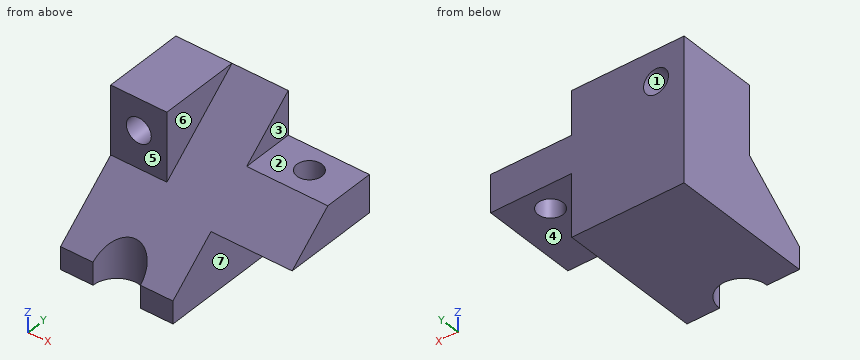
from build123d import *

# Parameters (mm, degrees)
F1_DEPTH = 77.5
F2_W     = 65
F2_H     = 35
F2_H_2   = 50
F3_DEPTH = 100
F4_R     = 19
F4_R_2   = 10
F5_DEPTH = 160.94138
F7_DEPTH = 45
F8_R     = 10
F9_DEPTH = 65


with BuildPart() as f1:
    # F0 (on Right) → F1 (new body, symmetric)
    with BuildSketch(Plane.YZ):
        Polygon((-57.5, 0), (57.5, 0), (57.5, 115), (-57.5, 18), align=None)
    extrude(amount=F1_DEPTH, both=True)

    # F2 (on Front) → F3 (cut, symmetric)
    with BuildSketch(Plane.XZ):
        with Locations((45, 97.5)):
            Rectangle(F2_W, F2_H)
        with Locations((45, 25)):
            Rectangle(F2_W, F2_H_2)
    extrude(amount=F3_DEPTH, both=True, mode=Mode.SUBTRACT)

    # F4 (on Top) → F5 (cut)
    with BuildSketch(Plane.XY):
        with Locations((-32.5, -57.5)):
            Circle(F4_R)
        with Locations((45.5, 37.5)):
            Circle(F4_R_2)
    extrude(amount=F5_DEPTH, mode=Mode.SUBTRACT)

    # F6 (on face) → F7 (join)
    with BuildSketch(Plane(origin=(-77.5, 0, 0), x_dir=(0, -1, 0), z_dir=(-1, 0, 0))):
        Polygon((7.5, 115), (-57.5, 115), (7.5, 60.1739130435), align=None)
    extrude(amount=-F7_DEPTH)

    # F8 (on face) → F9 (cut, through all)
    with BuildSketch(Plane.XZ.offset(7.5)):
        with Locations((-55, 90)):
            Circle(F8_R)
    extrude(amount=-F9_DEPTH, mode=Mode.SUBTRACT)


solid = f1.part
Input: part model. Units: mm. Frame: model coordinates. Face numbers are marked on the shaded views. A direction names the side the tool comes from. Coordinates: 2 decimals unless noted, no trailing zeros. Loops run counter-clockwise (first coordinate to the right, second up) from the corner with the lowest first, then second, coordinate; pieces in that order, holes last.
(1) Section A-A on x = -55. Return the cut outline in (y, z).
(2) Section D-D on x = 53.5. Return the cut outline in (y, z).
(3) Section C-C on z = 82.5. Return the cut outline in (x, y), then the cut area to 3 significant figures.
(4) Set-up query: the marked faces 5, 6 and 7. Return all of +Z, -Z, +X, -X, +Y, -Y with unobstructed straight access to the full face (end or side cutting, diameter ignored); none if empty.
(5) Section B-B on y = -51. Return the cut outline in (x, z).
(6) Material intervals for probe 1 along Z at (x, y) = (-55, 44.5); probe 2 along X at (y, z) = (37, 70); probe 3 along X at (y, z) = (24, 15.5), sorted ascending.
(7) Pull-direction query (Z, two-part tool) for the marked faces 1, 2, 3 and 4; classes: released by +Z, released by -Z, zero draft, split by the parting line, or undercut.
(8) First-contact query: pin 1 Ø13.5 at (x, z) = (-47.5, 77.5) entering from -Y; pin 2 Ø8 at (y, z) = (14, 11.5) entering from +X; pin 3 Ø16 at (x, z) = (-55, 90) entering from +Y; pin 4 Ø23 at (x, y) = (45.5, 37.5) entering from +Z. Flat tips, straight axial feed; report the tip coordinate or a pass-through.
Data:
1. outline: (-57.5, 0) - (57.5, 0) - (57.5, 80) - (-7.5, 80) - (-7.5, 60.17) - (-57.5, 18) - close; (-7.5, 100) - (57.5, 100) - (57.5, 115) - (-7.5, 115) - close
2. outline: (-19.56, 50) - (31.5, 50) - (31.5, 80) - (16.01, 80) - close; (43.5, 50) - (57.5, 50) - (57.5, 80) - (43.5, 80) - close
3. outline: (-77.5, -7.5) - (-61.61, -7.5) - (-61.61, 57.5) - (-77.5, 57.5) - close; (-48.39, -7.5) - (-32.5, -7.5) - (-32.5, 18.97) - (12.5, 18.97) - (12.5, 57.5) - (-48.39, 57.5) - close
3. area: 3,800 mm2
4. face 5: +Z, +X, -X, -Y
4. face 6: +Z, +X, -Y
4. face 7: -Z, +X, +Y, -Y
5. outline: (-77.5, 0) - (-50.35, 0) - (-50.35, 23.48) - (-77.5, 23.48) - close; (-14.65, 0) - (12.5, 0) - (12.5, 23.48) - (-14.65, 23.48) - close
6. probe 1: z = 0 to 80, 100 to 115
6. probe 2: x = -77.5 to 35.51, 55.49 to 77.5
6. probe 3: x = -77.5 to 12.5
7. face 1: undercut
7. face 2: released by +Z
7. face 3: zero draft
7. face 4: released by -Z
8. pin 1: stops at y = -7.5
8. pin 2: stops at x = 12.5
8. pin 3: passes through
8. pin 4: stops at z = 80
